from build123d import *

# Parameters (mm, degrees)
SKETCH1_W                               = 30
SKETCH1_H                               = 30
BOSS_EXTRUDE1_DEPTH                     = 10
FILLET1_R                               = 5
CBORE_FOR_M5_HEX_HEAD_BOLT2_D           = 4.5
CBORE_FOR_M5_HEX_HEAD_BOLT2_CBORE_D     = 5
CBORE_FOR_M5_HEX_HEAD_BOLT2_CBORE_DEPTH = 4.2
CBORE_FOR_M5_HEX_HEAD_BOLT1_D           = 4.5
CBORE_FOR_M5_HEX_HEAD_BOLT1_CBORE_D     = 5
CBORE_FOR_M5_HEX_HEAD_BOLT1_CBORE_DEPTH = 4.2
CUT_EXTRUDE1_DEPTH                      = 36


with BuildPart() as part:
    # Sketch1 → Boss-Extrude1 (new body)
    with BuildSketch(Plane(origin=(0, 0, 0), x_dir=(1, 0, 0), z_dir=(0, 1, 0))):
        Rectangle(SKETCH1_W, SKETCH1_H)
    extrude(amount=BOSS_EXTRUDE1_DEPTH)

    # Fillet1
    fillet1_edges = [part.edges().sort_by_distance(p)[0] for p in [
        (0, 0, -15),
        (0, 10, -15),
    ]]
    fillet(fillet1_edges, radius=FILLET1_R - 0.0001)  # a hair under: the kernel refuses the full size

    # CBORE for M5 Hex Head Bolt2 (through all)
    with Locations(Plane(origin=(15, 0, 0), x_dir=(0, 0, -1), z_dir=(1, 0, 0))):
        with Locations((10, 5)):
            cbore_for_m5_hex_head_bolt2 = CounterBoreHole(CBORE_FOR_M5_HEX_HEAD_BOLT2_D / 2, CBORE_FOR_M5_HEX_HEAD_BOLT2_CBORE_D / 2, CBORE_FOR_M5_HEX_HEAD_BOLT2_CBORE_DEPTH)

    # CBORE for M5 Hex Head Bolt1 (through all)
    with Locations(Plane(origin=(0, 10, 0), x_dir=(1, 0, 0), z_dir=(0, 1, 0))):
        with Locations((-10, -8), (10, -8), (0, 5)):
            CounterBoreHole(CBORE_FOR_M5_HEX_HEAD_BOLT1_D / 2, CBORE_FOR_M5_HEX_HEAD_BOLT1_CBORE_D / 2, CBORE_FOR_M5_HEX_HEAD_BOLT1_CBORE_DEPTH)

    # Sketch9 → Cut-Extrude1 (cut, through all)
    with BuildSketch(Plane(origin=(15, 0, 0), x_dir=(0, 0, -1), z_dir=(1, 0, 0))):
        with BuildLine():
            Line((-15, 10), (-15, 5))
            ThreePointArc((-15, 5), (-14.873403825, 7.51272405), (-14.494897428, 10))
            Line((-14.494897428, 10), (-15, 10))
        make_face()
        with BuildLine():
            Line((-15, 0), (-14.494897428, 0))
            ThreePointArc((-14.494897428, 0), (-14.873403825, 2.48727595), (-15, 5))
            Line((-15, 5), (-15, 0))
        make_face()
    extrude(amount=-CUT_EXTRUDE1_DEPTH, mode=Mode.SUBTRACT)

    # Mirror1: CBORE for M5 Hex Head Bolt2 across plane
    add(cbore_for_m5_hex_head_bolt2.mirror(Plane(origin=(0, 0, 0), x_dir=(0, 0, 1), z_dir=(1, 0, 0))), mode=Mode.SUBTRACT)


solid = part.part
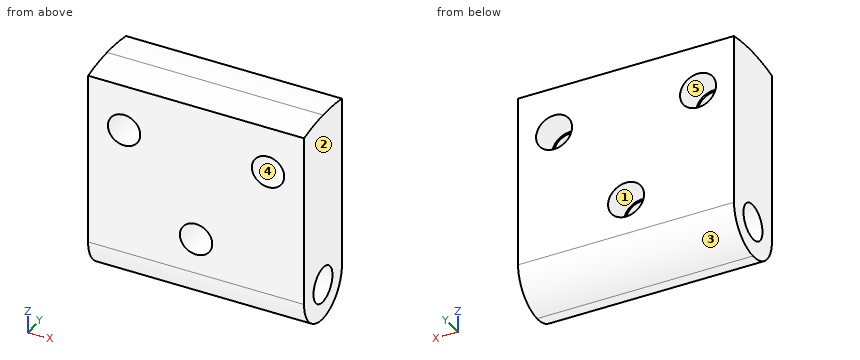
For this review, take the finished solid that the model builds, in its own axes (mm). Face numbers are marked on the shaded views. A direction names the side the tool comes from. Round coordinates to 2 decimals unless told otherwise and drop trailing zeros. Loops run counter-clockwise (first coordinate to the right, second up) from the corner with the lowest first, then second, coordinate; pieces in that order, holes last. Notation, with made-up numbers: (-22, 43) - (-9, 43) arc R26 ccw to (-9, 72) - close; hole circle Ø3 at (-24, 79). An arc over 180 degrees is marked (long way). One line per question, with ' | ' between items.
Q1. Take a section at C-C (y = 1.5). Give the boundary of the cut face in (x, z), and give its area (3 significant figures).
Taken from the geometry:
outline: (-15, -13.57) - (15, -13.57) - (15, 14.75) - (-15, 14.75) - close; hole circle Ø4.5 at (-10, 8); hole circle Ø4.5 at (0, -5); hole circle Ø4.5 at (10, 8) | area: 802 mm²
Q2. Take a section at B-B (z = -5). Give the boundary of the cut face in (x, y), and give its area (3 significant figures).
Taken from the geometry:
outline: (-15, 0) - (-2.25, 0) - (-2.25, 5.8) - (-2.5, 5.8) - (-2.5, 10) - (-15, 10) - close; (2.25, 0) - (15, 0) - (15, 10) - (2.5, 10) - (2.5, 5.8) - (2.25, 5.8) - close | area: 253 mm²
Q3. Take a section at A-A (x = -10). State how many separate pieces and enclosed holes the cut face has, and give its area (3 significant figures).
Taken from the geometry:
separate pieces: 2 | enclosed holes: 1 | area: 225 mm²
Q4. For line 1 along Y through (x, z) = (-3.5, -10); line 2 along Z through (x, y) = (-1.75, 7); line 3 along Z through (x, y) = (9.5, 4.75), list the stretches that pass through material, from the lowest coordinate up. Write a range as [from, to].
Taken from the geometry:
line 1: y = [0, 2.75], [7.25, 10] | line 2: z = [-14.58, -11.03], [-8.97, -6.79], [-3.21, 14.92] | line 3: z = [-14.99, -12.24], [-7.76, 5.81], [10.19, 15]
Q5. Tool access review of the marked faces 4 and 5: name each direction out of +Z, -Z, +X, -X, +Y, -Y from which nothing blocks a thin tool from reaching the whole face with its end or side.
Taken from the geometry:
face 4: +Y, -Y | face 5: +Y
Q6. The part is to be moulded in two halves that separate along Z. For the marked faces 1, 2 and 3, say which applies: released by +Z, released by -Z, zero draft, split by the parting line, or undercut.
Taken from the geometry:
face 1: undercut | face 2: zero draft | face 3: released by -Z
Q7. For pin 1 (1 mm diameter, centred on x = -0.5, y = 6.5, fed in from -Z); pin 2 (1 mm diameter, centred on x = -10, y = 6, fed in from -Z); pin 3 (2.5 mm diameter, centred on y = 4.5, z = -11, fed in from -X), all flat-tipped, find the tip position at first contact; note any pin that passes through.
Taken from the geometry:
pin 1: stops at z = -14.9 | pin 2: stops at z = -14.97 | pin 3: stops at x = -10.8
Q8. Take a section at D-D (y = 4). Give the boundary of the cut face in (x, z), and give its area (3 significant figures).
Taken from the geometry:
outline: (-15, -14.9) - (15, -14.9) - (15, -12.29) - (10.8, -12.29) - (10.8, -12.02) - (-10.8, -12.02) - (-10.8, -12.29) - (-15, -12.29) - close; (-15, -7.71) - (-10.8, -7.71) - (-10.8, -7.98) - (10.8, -7.98) - (10.8, -7.71) - (15, -7.71) - (15, 14.98) - (-15, 14.98) - close; hole circle Ø4.5 at (-10, 8); hole circle Ø4.5 at (0, -5); hole circle Ø4.5 at (10, 8) | area: 723 mm²
